Print and shaded views of the part. All mm, measured from the part's lowest x, y and z. A direction names the side the tool comes from. Round coordinates to 2 decimals unless told otherwise and drop trailing zeros. Order: outer loops, then holes, each group sorted by start corner. A loop starts at its lowest first (then second) coordinate and runs counter-clockwise, first axis right, second up. Notation, with made-up numbers: (-4, 79) - (51, 79) arc R22 ccw to (51, 87) - close; hole circle Ø9 at (41, 2.5). An arc over 180 degrees is marked (long way). Write item = value, one per line.
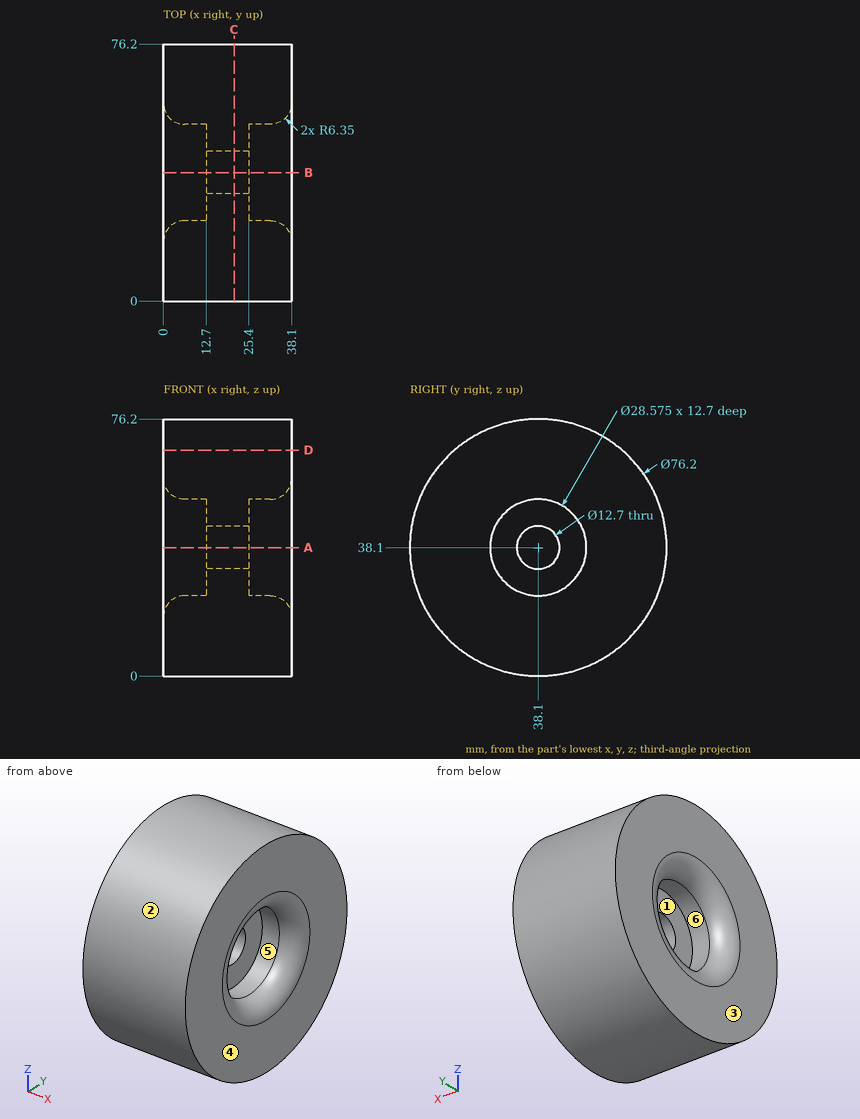
(1) Tool access for the marked faces 4, 5 and 6: list every direction of +Z, -Z, +X, -X, +Y, -Y with a clear straight run to the whole face (end or side of a thin tool).
Solved:
face_4 = +Z, -Z, +X, +Y, -Y
face_5 = +X
face_6 = -X
(2) Pull direction Y, two halves, no side cores. Call the marked faces 1, 2 and 3: released by +Y, released by -Y, zero draft, split by the parting line, or undercut.
Solved:
face_1 = undercut
face_2 = split by the parting line
face_3 = zero draft
(3) Band-saw the part on C-C on x = 21. List the corners of the cut face in (y, z), plus the area to 3 significant figures.
Solved:
outline = circle Ø76.2 at (38.1, 38.1); hole circle Ø12.7 at (38.1, 38.1)
area = 4,430 mm²
(4) Probe line 1 along Z through (x, y) = (11.75, 38.1); line 2 along Y through (x, z) = (16, 38). List the from-to ranges inside material, lowest first.
Solved:
line_1 = 0 to 23.81, 52.39 to 76.2
line_2 = 0 to 31.75, 44.45 to 76.2
(5) Band-saw the part on D-D on z = 67. List the corners of the cut face in (x, y), plus the area to 3 significant figures.
Solved:
outline = (0, 13.27) - (38.1, 13.27) - (38.1, 62.93) - (0, 62.93) - close
area = 1,890 mm²
(6) Band-saw the part on A-A on z = 38.1. List the corners of the cut face in (x, y).
Solved:
outline = (0, 0) - (38.1, 0) - (38.1, 17.46) arc R6.35 ccw to (31.75, 23.81) - (25.4, 23.81) - (25.4, 31.75) - (12.7, 31.75) - (12.7, 23.81) - (6.35, 23.81) arc R6.35 ccw to (0, 17.46) - close; (0, 58.74) arc R6.35 ccw to (6.35, 52.39) - (12.7, 52.39) - (12.7, 44.45) - (25.4, 44.45) - (25.4, 52.39) - (31.75, 52.39) arc R6.35 ccw to (38.1, 58.74) - (38.1, 76.2) - (0, 76.2) - close
(7) Drop flat-ended pins along their axis: pin 1 (23 mm diameter, centred on y = 38.1, z = 38.1, fed in from -X); pin 2 (6 mm diameter, centred on x = 29.5, z = 22.5, fed in from -Y); pin 3 (5 mm diameter, centred on x = 13.5, z = 43.5, fed in from -Y); pin 4 (10 mm diameter, centred on y = 38.1, z = 38.1, fed in from +X). Give the stop position or say it passes through.
Solved:
pin_1 = 12.7
pin_2 = 2.14
pin_3 = 0.11
pin_4 = through
